Work out the finished part from the listing and answer in its coordinate system (mm). Face numbers are marked on the shaded views. Give positions to 0.01 mm unless a question says otherwise; leave off trailing zeros. Order: outer loops, then holes, each group sorted by start corner. A loop starts at its lowest first (then second) coordinate and runs counter-clockwise, first axis right, second up.
```python
from build123d import *

# Parameters (mm, degrees)
SKETCH1_R           = 38.1
BOSS_EXTRUDE2_DEPTH = 50.8
SKETCH3_R           = 15.875
CUT_EXTRUDE2_DEPTH  = 47.752
SKETCH3_6_R         = 33.147
SKETCH3_6_R_2       = 15.875
CUT_EXTRUDE3_DEPTH  = 25.4
SKETCH4_R           = 9.525
CUT_EXTRUDE4_DEPTH  = 3.048


with BuildPart() as part:
    # Sketch1 → Boss-Extrude2 (new body)
    with BuildSketch(Plane(origin=(0, 0, 0), x_dir=(1, 0, 0), z_dir=(0, 1, 0))):
        Circle(SKETCH1_R)
    extrude(amount=BOSS_EXTRUDE2_DEPTH)

    # Sketch3 → Cut-Extrude2 (cut)
    with BuildSketch(Plane(origin=(0, 50.8, 0), x_dir=(1, 0, 0), z_dir=(0, 1, 0))):
        Circle(SKETCH3_R)
    extrude(amount=-CUT_EXTRUDE2_DEPTH, mode=Mode.SUBTRACT)

    # Sketch3<6> → Cut-Extrude3 (cut)
    with BuildSketch(Plane(origin=(0, 50.8, 0), x_dir=(1, 0, 0), z_dir=(0, 1, 0))):
        Circle(SKETCH3_6_R)
        Circle(SKETCH3_6_R_2, mode=Mode.SUBTRACT)
    extrude(amount=-CUT_EXTRUDE3_DEPTH, mode=Mode.SUBTRACT)

    # Sketch4 → Cut-Extrude4 (cut)
    with BuildSketch(Plane(origin=(0, 0, 0), x_dir=(-1, 0, 0), z_dir=(0, -1, 0))):
        Circle(SKETCH4_R)
    extrude(amount=-CUT_EXTRUDE4_DEPTH, mode=Mode.SUBTRACT)


solid = part.part
```
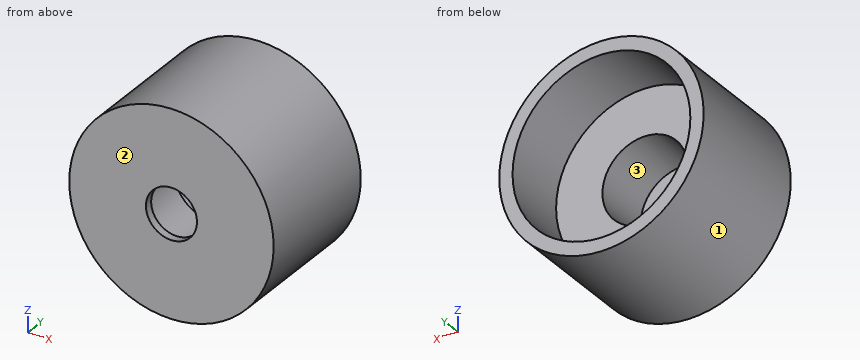
1. Straight lines are drawn through the part: probe 1 along X at (y, z) = (45.25, 0); probe 2 along Z at (x, y) = (0, 16) (3 decimals); probe 3 along Z at (x, y) = (0, 2) (3 decimals). For each, find the intervals that lie inside material, in ascending order.
Findings below:
probe 1: x = -38.1 to -33.15, 33.15 to 38.1
probe 2: z = -38.1 to -15.875, 15.875 to 38.1
probe 3: z = -38.1 to -9.525, 9.525 to 38.1
2. Given P1, Ø8, axis at x = -6.5, y = 8, coming from the -Z side; P2, Ø6, axis at x = -6.5, y = 12.5, coming from the -Z side; P3, Ø10, axis at x = -7, y = 18.5, coming from the +Z side; P4, Ø6, axis at x = 2, z = -11, coming from the -Y side, each flat-ended and moving along its own axis, determine where each tip first touches the part or whether it passes through.
Findings below:
P1: stops at z = -38.02
P2: stops at z = -37.94
P3: stops at z = 38.05
P4: stops at y = 0
3. The part is cut by section C-C (x = -12.5). Write down the section's boundary in (y, z).
Findings below:
outline: (0, -35.99) - (50.8, -35.99) - (50.8, -30.7) - (25.4, -30.7) - (25.4, -9.79) - (3.05, -9.79) - (3.05, 9.79) - (25.4, 9.79) - (25.4, 30.7) - (50.8, 30.7) - (50.8, 35.99) - (0, 35.99) - close
4. The part is cut by section D-D (z = -10.5). Write down the section's boundary in (x, y), then the cut area to 3 significant figures.
Findings below:
outline: (-36.62, 0) - (36.62, 0) - (36.62, 50.8) - (31.44, 50.8) - (31.44, 25.4) - (11.91, 25.4) - (11.91, 3.05) - (-11.91, 3.05) - (-11.91, 25.4) - (-31.44, 25.4) - (-31.44, 50.8) - (-36.62, 50.8) - close
area: 1,590 mm2
5. The mould has two halves that part along Z. Classify the marked faces 1, 2 and 3: pulls with the +Z half, pulls with the -Z half, needs draft (parallel to the pull), parting line crosses it, or undercut.
Findings below:
face 1: parting line crosses it
face 2: needs draft
face 3: undercut
6. The part is cut by section A-A (x = 0). Write down the section's boundary in (y, z) (3 decimals), then the cut area to 3 significant figures.
Findings below:
outline: (0, -38.1) - (50.8, -38.1) - (50.8, -33.147) - (25.4, -33.147) - (25.4, -15.875) - (3.048, -15.875) - (3.048, -9.525) - (0, -9.525) - close; (0, 9.525) - (3.048, 9.525) - (3.048, 15.875) - (25.4, 15.875) - (25.4, 33.147) - (50.8, 33.147) - (50.8, 38.1) - (0, 38.1) - close
area: 1,420 mm2
7. The part is cut by section B-B (z = 0). Write down the section's boundary in (x, y) (3 decimals).
Findings below:
outline: (-38.1, 0) - (-9.525, 0) - (-9.525, 3.048) - (-15.875, 3.048) - (-15.875, 25.4) - (-33.147, 25.4) - (-33.147, 50.8) - (-38.1, 50.8) - close; (9.525, 0) - (38.1, 0) - (38.1, 50.8) - (33.147, 50.8) - (33.147, 25.4) - (15.875, 25.4) - (15.875, 3.048) - (9.525, 3.048) - close
